Geometry: see drawing. Coordinates: mm, zero at the bounding-box minimum. A direction names the side the tool comes from. Round coordinates to 2 decimals unless told otherwise and drop trailing zeros. Write each loop counter-clockwise with the first axis right and the second up, starting at its lowest first coordinate (ties: lowest second). Pieces come first, ordered by that corner, then holes. Notation, with made-up numbers: (-24.75, 61) - (24.25, 61) arc R23 ccw to (24.25, 76) - close; hole circle Ø2 at (59, 32.25). An arc over 180 degrees is marked (long way). Use a Markdown table: item, result. Add a question column.
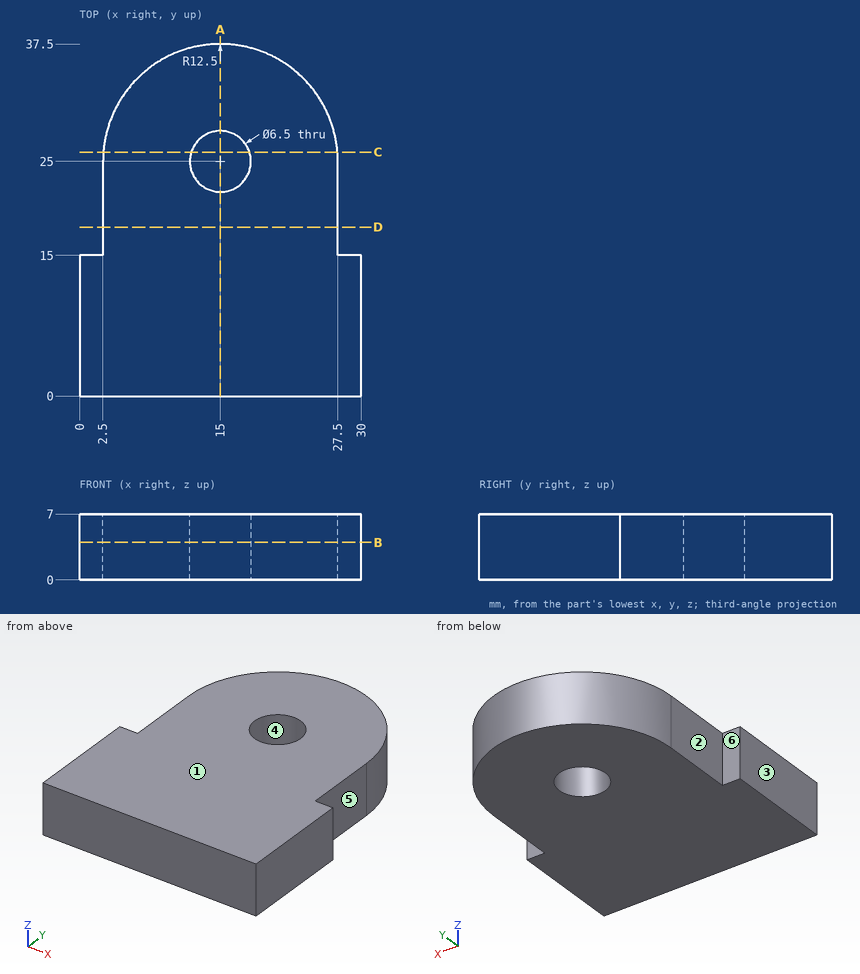
1) Pin query (flat end, axial travel): P1, Ø0.8, axis at x = 29, z = 3.5, coming from the +Y side; P2, Ø6, axis at x = 16.5, y = 5, coming from the -Z side; P3, Ø3, axis at x = 12, z = 6, coming from the +Y side; P4, Ø3, axis at y = 19.5, z = 1, coming from the +X side. Return the tip coordinate at first contact, or that it passes through.
2) Section A-A, the plane x = 15. Return the cut outline in (y, z).
3) Material intervals for L1, parallel to Y at x = 15, z = 3; L2, parallel to X at y = 16, z = 6.5; L3, parallel to X at y = 27, z = 4.5, sorted ascending. Write a range as from..to.
4) Section C-C, the plane y = 26. Return the cut outline in (x, z).
5) Set-up query: the marked faces 1 and 2. Return all of +Z, -Z, +X, -X, +Y, -Y with unobstructed straight access to the full face (end or side cutting, diameter ignored); none if empty.
6) Section B-B, the plane z = 4. Return the cut outline in (x, y), then the cut area to 3 significant figures.
7) Draft query along X for the marked faces 3, 4, 5 and 6. Return one class per face: released by +X, released by -X, zero draft, split by the parting line, or undercut.
8) Section D-D, the plane y = 18. Return the cut outline in (x, z).
Output values:
| question | item | result |
|---|---|---|
| 1 | P1 | stops at y = 15 |
| 1 | P2 | stops at z = 0 |
| 1 | P3 | stops at y = 37.41 |
| 1 | P4 | stops at x = 27.5 |
| 2 | outline | (0, 0) - (21.75, 0) - (21.75, 7) - (0, 7) - close; (28.25, 0) - (37.5, 0) - (37.5, 7) - (28.25, 7) - close |
| 3 | L1 | y = 0..21.75, 28.25..37.5 |
| 3 | L2 | x = 2.5..27.5 |
| 3 | L3 | x = 2.66..12.44, 17.56..27.34 |
| 4 | outline | (2.54, 0) - (11.91, 0) - (11.91, 7) - (2.54, 7) - close; (18.09, 0) - (27.46, 0) - (27.46, 7) - (18.09, 7) - close |
| 5 | face 1 | +Z, +X, -X, +Y, -Y |
| 5 | face 2 | +Z, -Z, -X, +Y |
| 6 | outline | (0, 0) - (30, 0) - (30, 15) - (27.5, 15) - (27.5, 25) arc R12.5 ccw to (2.5, 25) - (2.5, 15) - (0, 15) - close; hole circle Ø6.5 at (15, 25) |
| 6 | area | 912 mm^2 |
| 7 | face 3 | released by -X |
| 7 | face 4 | undercut |
| 7 | face 5 | released by +X |
| 7 | face 6 | zero draft |
| 8 | outline | (2.5, 0) - (27.5, 0) - (27.5, 7) - (2.5, 7) - close |
